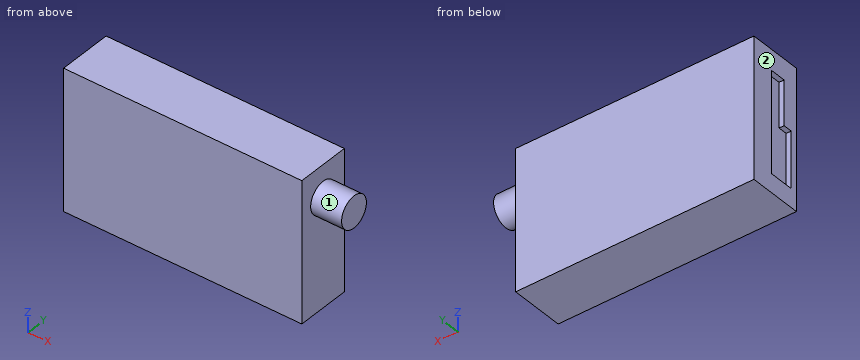
from build123d import *

# Parameters (mm, degrees)
SKETCH1_W           = 47.36
SKETCH1_H           = 27.9
BOSS_EXTRUDE1_DEPTH = 5.35
SKETCH2_R           = 3.125
BOSS_EXTRUDE2_DEPTH = 6.15
SKETCH3_W           = 11.2
SKETCH3_H           = 5
CUT_EXTRUDE1_DEPTH  = 1
SKETCH5_W           = 8.9
SKETCH5_H           = 3.2
CUT_EXTRUDE2_DEPTH  = 1


with BuildPart() as part:
    # Sketch1 → Boss-Extrude1 (new, symmetric)
    with BuildSketch(Plane(origin=(0, 0, 0), x_dir=(1, 0, 0), z_dir=(0, 1, 0))):
        Rectangle(SKETCH1_W, SKETCH1_H)
    extrude(amount=BOSS_EXTRUDE1_DEPTH, both=True)

    # Sketch2 → Boss-Extrude2 (add)
    with BuildSketch(Plane(origin=(23.68, 0, 0), x_dir=(0, 0, -1), z_dir=(1, 0, 0))):
        with Locations(Location((-7.575, 0, 0), (0, 0, 180))):
            Circle(SKETCH2_R)
    extrude(amount=BOSS_EXTRUDE2_DEPTH)

    # Sketch3 → Cut-Extrude1 (cut)
    with BuildSketch(Plane.ZY.offset(23.68)):
        with Locations((-4.65, -1.55)):
            Rectangle(SKETCH3_W, SKETCH3_H)
    extrude(amount=-CUT_EXTRUDE1_DEPTH, mode=Mode.SUBTRACT)

    # Sketch5 → Cut-Extrude2 (cut)
    with BuildSketch(Plane.ZY.offset(23.68)):
        with Locations((5.4, -0.65)):
            Rectangle(SKETCH5_W, SKETCH5_H)
    extrude(amount=-CUT_EXTRUDE2_DEPTH, mode=Mode.SUBTRACT)


solid = part.part
Can you work these out from the model? Positions are in its coordinate system, mm. Face numbers are marked on the shaded views. A direction names the side the tool comes from. Give positions to 0.01 mm unless a question says otherwise; leave off trailing zeros. Order: outer loops, then holes, each group sorted by start corner. A loop starts at its lowest first (then second) coordinate and runs counter-clockwise, first axis right, second up. Notation, with made-up numbers: M -3.5,6.5 L 4.5,6.5 A35 ccw 4.5,44.5 Z; hole C 1,24 d7. An arc over 180 degrees is marked long. Use a Markdown table: item, result. Add a question column.
Item 1: For the marked faces 1 and 2, which set-ups out of +Z, -Z, +X, -X, +Y, -Y let a thin tool reach every point of the face, with its end or its side?
Item 2: Suppose I cut it at D-D (z = 11.5). List the corners of the cut face in (x, y) for me, then the cut area to 3 significant figures.
Item 3: Suppose I cut it at B-B (y = 0). List the corners of the cut face in (x, z) for me.
Item 4: Will these pins go through, and if not, where does the flat tip stop? pin 1 (2.5 mm diameter, centred on y = -1.5, z = -2, fed in from -X); pin 2 (1.5 mm diameter, centred on y = -3, z = -2.5, fed in from +X).
Item 5: Suppose I cut it at C-C (z = -0.5). List the corners of the cut face in (x, y) for me.
Item 6: If I drill on L1, parallel to X at y = -4.5, z = 9; L2, parallel to X at y = -3.5, z = -2.5; L3, parallel to Z at x = 27, y = 2.5, over which ranges is the centre line in solid material (lowest first)? Write a range as [from, to].
Item 7: Suppose I cut it at A-A (z = 3). List the corners of the cut face in (x, y) for me.
Answer sheet:
| question | item | result |
|---|---|---|
| 1 | face 1 | +X |
| 1 | face 2 | +Z, -Z, -X, +Y, -Y |
| 2 | outline | M -23.68,-5.35 L 23.68,-5.35 L 23.68,5.35 L -23.68,5.35 Z |
| 2 | area | 507 mm² |
| 3 | outline | M -23.68,-13.95 L 23.68,-13.95 L 23.68,4.45 L 29.83,4.45 L 29.83,10.7 L 23.68,10.7 L 23.68,13.95 L -23.68,13.95 L -23.68,9.85 L -22.68,9.85 L -22.68,-10.25 L -23.68,-10.25 Z |
| 4 | pin 1 | stops at x = -22.68 |
| 4 | pin 2 | stops at x = 23.68 |
| 5 | outline | M -23.68,-5.35 L 23.68,-5.35 L 23.68,5.35 L -23.68,5.35 L -23.68,0.95 L -22.68,0.95 L -22.68,-4.05 L -23.68,-4.05 Z |
| 6 | L1 | x = [-23.68, 23.68] |
| 6 | L2 | x = [-22.68, 23.68] |
| 6 | L3 | z = [5.7, 9.45] |
| 7 | outline | M -23.68,-5.35 L 23.68,-5.35 L 23.68,5.35 L -23.68,5.35 L -23.68,0.95 L -22.68,0.95 L -22.68,-2.25 L -23.68,-2.25 Z |
